The model under review builds one solid part; all positions refer to its coordinate system, in mm. A direction names the side the tool comes from. Coordinates: 2 decimals unless noted, no trailing zeros. Order: outer loops, then holes, each group sorted by start corner. A loop starts at its lowest first (then second) coordinate and runs counter-clockwise, first axis right, second up.
```python
from build123d import *

# Parameters (mm, degrees)
F1_DEPTH = 1.7145
F0_R     = 9.525
F2_DEPTH = 3.175
F3_R     = 6.35
F4_R     = 5.08


with BuildPart() as f1:
    # F0 (on Top) → F1 (new body)
    with BuildSketch(Plane.XY):
        with BuildLine():
            ThreePointArc((23.9050999455, -6.4692674698), (24.5490837421, -3.2630832697), (24.765, 0))
            ThreePointArc((24.765, 0), (19.6285885254, 15.1004548773), (6.35, 23.9370575677))
            ThreePointArc((6.35, 23.9370575677), (4.2391432725, 24.3994854314), (2.0960107473, 24.6761415936))
            ThreePointArc((2.0960107473, 24.6761415936), (2.1906494626, 24.3119724675), (2.2225, 23.9370575677))
            ThreePointArc((2.2225, 23.9370575677), (-0.3749148998, 21.7464081051), (-2.0960107473, 24.6761415936))
            ThreePointArc((-2.0960107473, 24.6761415936), (-4.2391432725, 24.3994854314), (-6.35, 23.9370575677))
            ThreePointArc((-6.35, 23.9370575677), (-21.4471191247, 12.3825), (-23.9050999455, -6.4692674698))
            ThreePointArc((-23.9050999455, -6.4692674698), (-23.2501458591, -8.5285369514), (-22.4181708611, -10.5228722431))
            ThreePointArc((-22.4181708611, -10.5228722431), (-19.9594610417, -9.8839132486), (-18.5075999455, -11.9685287839))
            ThreePointArc((-18.5075999455, -11.9685287839), (-19.02039931, -13.3885393426), (-20.3221601138, -14.1532693505))
            ThreePointArc((-20.3221601138, -14.1532693505), (-19.0110025866, -15.87094848), (-17.5550999455, -17.4677900979))
            ThreePointArc((-17.5550999455, -17.4677900979), (0, -24.765), (17.5550999455, -17.4677900979))
            ThreePointArc((17.5550999455, -17.4677900979), (19.0110025866, -15.87094848), (20.3221601138, -14.1532693505))
            ThreePointArc((20.3221601138, -14.1532693505), (18.8053584856, -10.8572787839), (22.4181708611, -10.5228722431))
            ThreePointArc((22.4181708611, -10.5228722431), (23.2501458591, -8.5285369514), (23.9050999455, -6.4692674698))
        make_face()
        with BuildLine():
            ThreePointArc((-6.35, -11.7260276735), (-6.8244038201, 11.4564277809), (13.335, 0))
            ThreePointArc((13.335, 0), (11.4564277809, -6.8244038201), (6.35, -11.7260276735))
            Line((6.35, -11.7260276735), (6.35, -20.955))
            Line((6.35, -20.955), (-6.35, -20.955))
            Line((-6.35, -20.955), (-6.35, -11.7260276735))
        make_face(mode=Mode.SUBTRACT)
        with BuildLine():
            ThreePointArc((2.0960107473, 24.6761415936), (4.2391432725, 24.3994854314), (6.35, 23.9370575677))
            ThreePointArc((6.35, 23.9370575677), (0, 30.2870575677), (-6.35, 23.9370575677))
            ThreePointArc((-6.35, 23.9370575677), (-4.2391432725, 24.3994854314), (-2.0960107473, 24.6761415936))
            ThreePointArc((-2.0960107473, 24.6761415936), (0, 26.1595575677), (2.0960107473, 24.6761415936))
        make_face()
        with BuildLine():
            ThreePointArc((17.5550999455, -17.4677900979), (26.2293612595, -15.1435287839), (23.9050999455, -6.4692674698))
            ThreePointArc((23.9050999455, -6.4692674698), (23.2501458591, -8.5285369514), (22.4181708611, -10.5228722431))
            ThreePointArc((22.4181708611, -10.5228722431), (22.8147154808, -11.1978898801), (22.9525999455, -11.9685287839))
            ThreePointArc((22.9525999455, -11.9685287839), (22.1501105043, -13.6782294193), (20.3221601138, -14.1532693505))
            ThreePointArc((20.3221601138, -14.1532693505), (19.0110025866, -15.87094848), (17.5550999455, -17.4677900979))
        make_face()
        with BuildLine():
            ThreePointArc((-22.4181708611, -10.5228722431), (-23.2501458591, -8.5285369514), (-23.9050999455, -6.4692674698))
            ThreePointArc((-23.9050999455, -6.4692674698), (-26.2293612595, -15.1435287839), (-17.5550999455, -17.4677900979))
            ThreePointArc((-17.5550999455, -17.4677900979), (-19.0110025866, -15.87094848), (-20.3221601138, -14.1532693505))
            ThreePointArc((-20.3221601138, -14.1532693505), (-22.6548414054, -13.0797787839), (-22.4181708611, -10.5228722431))
        make_face()
    extrude(amount=-F1_DEPTH)

    # F0 (on Top) → F2 (join)
    with BuildSketch(Plane.XY):
        with BuildLine():
            ThreePointArc((23.9050999455, -6.4692674698), (24.5490837421, -3.2630832697), (24.765, 0))
            ThreePointArc((24.765, 0), (19.6285885254, 15.1004548773), (6.35, 23.9370575677))
            ThreePointArc((6.35, 23.9370575677), (4.2391432725, 24.3994854314), (2.0960107473, 24.6761415936))
            ThreePointArc((2.0960107473, 24.6761415936), (2.1906494626, 24.3119724675), (2.2225, 23.9370575677))
            ThreePointArc((2.2225, 23.9370575677), (-0.3749148998, 21.7464081051), (-2.0960107473, 24.6761415936))
            ThreePointArc((-2.0960107473, 24.6761415936), (-4.2391432725, 24.3994854314), (-6.35, 23.9370575677))
            ThreePointArc((-6.35, 23.9370575677), (-21.4471191247, 12.3825), (-23.9050999455, -6.4692674698))
            ThreePointArc((-23.9050999455, -6.4692674698), (-23.2501458591, -8.5285369514), (-22.4181708611, -10.5228722431))
            ThreePointArc((-22.4181708611, -10.5228722431), (-19.9594610417, -9.8839132486), (-18.5075999455, -11.9685287839))
            ThreePointArc((-18.5075999455, -11.9685287839), (-19.02039931, -13.3885393426), (-20.3221601138, -14.1532693505))
            ThreePointArc((-20.3221601138, -14.1532693505), (-19.0110025866, -15.87094848), (-17.5550999455, -17.4677900979))
            ThreePointArc((-17.5550999455, -17.4677900979), (0, -24.765), (17.5550999455, -17.4677900979))
            ThreePointArc((17.5550999455, -17.4677900979), (19.0110025866, -15.87094848), (20.3221601138, -14.1532693505))
            ThreePointArc((20.3221601138, -14.1532693505), (18.8053584856, -10.8572787839), (22.4181708611, -10.5228722431))
            ThreePointArc((22.4181708611, -10.5228722431), (23.2501458591, -8.5285369514), (23.9050999455, -6.4692674698))
        make_face()
        with BuildLine():
            ThreePointArc((-6.35, -11.7260276735), (-6.8244038201, 11.4564277809), (13.335, 0))
            ThreePointArc((13.335, 0), (11.4564277809, -6.8244038201), (6.35, -11.7260276735))
            Line((6.35, -11.7260276735), (6.35, -20.955))
            Line((6.35, -20.955), (-6.35, -20.955))
            Line((-6.35, -20.955), (-6.35, -11.7260276735))
        make_face(mode=Mode.SUBTRACT)
        with BuildLine():
            ThreePointArc((6.35, -11.7260276735), (11.4564277809, -6.8244038201), (13.335, 0))
            ThreePointArc((13.335, 0), (-6.8244038201, 11.4564277809), (-6.35, -11.7260276735))
            ThreePointArc((-6.35, -11.7260276735), (0, -13.335), (6.35, -11.7260276735))
        make_face()
        Circle(F0_R, mode=Mode.SUBTRACT)
        with BuildLine():
            ThreePointArc((6.35, -11.7260276735), (0, -13.335), (-6.35, -11.7260276735))
            Line((-6.35, -11.7260276735), (-6.35, -20.955))
            Line((-6.35, -20.955), (6.35, -20.955))
            Line((6.35, -20.955), (6.35, -11.7260276735))
        make_face()
        with BuildLine():
            ThreePointArc((2.0960107473, 24.6761415936), (4.2391432725, 24.3994854314), (6.35, 23.9370575677))
            ThreePointArc((6.35, 23.9370575677), (0, 30.2870575677), (-6.35, 23.9370575677))
            ThreePointArc((-6.35, 23.9370575677), (-4.2391432725, 24.3994854314), (-2.0960107473, 24.6761415936))
            ThreePointArc((-2.0960107473, 24.6761415936), (0, 26.1595575677), (2.0960107473, 24.6761415936))
        make_face()
        with BuildLine():
            ThreePointArc((-22.4181708611, -10.5228722431), (-23.2501458591, -8.5285369514), (-23.9050999455, -6.4692674698))
            ThreePointArc((-23.9050999455, -6.4692674698), (-26.2293612595, -15.1435287839), (-17.5550999455, -17.4677900979))
            ThreePointArc((-17.5550999455, -17.4677900979), (-19.0110025866, -15.87094848), (-20.3221601138, -14.1532693505))
            ThreePointArc((-20.3221601138, -14.1532693505), (-22.6548414054, -13.0797787839), (-22.4181708611, -10.5228722431))
        make_face()
        with BuildLine():
            ThreePointArc((17.5550999455, -17.4677900979), (26.2293612595, -15.1435287839), (23.9050999455, -6.4692674698))
            ThreePointArc((23.9050999455, -6.4692674698), (23.2501458591, -8.5285369514), (22.4181708611, -10.5228722431))
            ThreePointArc((22.4181708611, -10.5228722431), (22.8147154808, -11.1978898801), (22.9525999455, -11.9685287839))
            ThreePointArc((22.9525999455, -11.9685287839), (22.1501105043, -13.6782294193), (20.3221601138, -14.1532693505))
            ThreePointArc((20.3221601138, -14.1532693505), (19.0110025866, -15.87094848), (17.5550999455, -17.4677900979))
        make_face()
    extrude(amount=F2_DEPTH)

    # F3
    f3_edges = [f1.edges().sort_by_distance(p)[0] for p in [
        (-23.9051, -6.469267, -0.85725),
        (6.35, 23.937058, 0.73025),
        (17.5551, -17.46779, 0.73025),
        (23.9051, -6.469267, 0.73025),
        (-17.5551, -17.46779, -0.85725),
        (-17.5551, -17.46779, 1.5875),
        (-23.9051, -6.469267, 1.5875),
        (-6.35, 23.937058, 1.5875),
        (-6.35, 23.937058, -0.85725),
    ]]
    fillet(f3_edges, radius=F3_R)

    # F4
    f4_edges = [f1.edges().sort_by_distance(p)[0] for p in [
        (-6.35, -11.726028, -0.85725),
        (6.35, -11.726028, -0.85725),
        (6.35, -20.955, -0.85725),
        (-6.35, -20.955, -0.85725),
    ]]
    fillet(f4_edges, radius=F4_R)


solid = f1.part
```
(1) Draft analysis for pull direction Y (two halves, no side actions). For faces 3 (the face through (26.18, -15.23, 0.7)), 4 (the face through (12, -9, -1.714)), 5 (the face through (-6.35, -15, -1)), state which applies: released by +Y, released by -Y, zero draft, split by the parting line, or undercut.
A:
face 3: split by the parting line
face 4: zero draft
face 5: undercut
(2) We need section B-B, the plane x = -21.5. Write out the cut boundary in (y, z) (1 decimal), and give its area (3 significant figures).
A:
outline: (-18.3, -1.7) - (-14.1, -1.7) - (-14.1, 3.2) - (-18.3, 3.2) - close; (-9.9, -1.7) - (12.3, -1.7) - (12.3, 3.2) - (-9.9, 3.2) - close
area: 129 mm2
(3) We need section A-A, the plane x = 0. Write out the cut boundary in (y, z) (1 decimal).
A:
outline: (-24.8, -1.7) - (-21, -1.7) - (-21, 0) - (-9.5, 0) - (-9.5, 3.2) - (-24.8, 3.2) - close; (9.5, 0) - (13.3, 0) - (13.3, -1.7) - (21.7, -1.7) - (21.7, 3.2) - (9.5, 3.2) - close; (26.2, -1.7) - (30.3, -1.7) - (30.3, 3.2) - (26.2, 3.2) - close
(4) Machinability: for faces 1 (the face through (0, -20.955, -1)), 2 (the face through (0.105, 30.286, 0.696)), which of the approach directions +Z, -Z, +X, -X, +Y, -Y give a long, thin tool a straight path to every point of the face, cutting with its end or side? Answer none if there is none.
A:
face 1: -Z
face 2: +Z, -Z, +Y
(5) We need section D-D, the plane x = 12. Write out the cut boundary in (y, z) (1 decimal), and give its area (3 significant figures).
A:
outline: (-21.7, -1.7) - (-5.8, -1.7) - (-5.8, 0) - (5.8, 0) - (5.8, -1.7) - (21.7, -1.7) - (21.7, 3.2) - (-21.7, 3.2) - close
area: 192 mm2
(6) For pin 1 Ø7 at (x, y) = (20.73, -11.97) entering from +Z (3 decimals); pin 2 Ø0.7 at (y, z) = (-15, -1) entering from -X; pin 3 Ø0.5 at (x, z) = (-0.5, -1) entering from +Y; pin 4 Ø21.5 at (x, y) = (0, 0) entering from -Z, all flat-tipped, find the tip position at first contact; note any pin that passes through.
A:
pin 1: stops at z = 3.175
pin 2: stops at x = -26.49
pin 3: stops at y = 30.28
pin 4: stops at z = 0
(7) We need section C-C, the plane y = 14. Write out the cut boundary in (x, z) (1 decimal).
A:
outline: (-20.4, -1.7) - (20.4, -1.7) - (20.4, 3.2) - (-20.4, 3.2) - close
(8) Wall thickness on probe 1 along Y at (x, z) = (0, 1.1) (3 decimals); probe 2 along Y at (x, z) = (0, -0.35) (3 decimals); probe 3 along X at (y, z) = (-12.5, -1.05): over which ranges is each line inside the solid? List them lowest first.
A:
probe 1: y = -24.765 to -9.525, 9.525 to 21.715, 26.16 to 30.287
probe 2: y = -24.765 to -20.955, 13.335 to 21.715, 26.16 to 30.287
probe 3: x = -27.06 to -22.89, -18.57 to -6.73, 6.73 to 18.57, 22.89 to 27.06
